Could you check a few things on this model? Use its own coordinates, in mm. Round coordinates to 2 decimals unless told otherwise and drop trailing zeros. Loops run counter-clockwise (first coordinate to the right, second up) from the corner with the lowest first, then second, coordinate; pieces in that order, holes last. Notation, with made-up numbers: (31.5, 44.25) - (63.5, 44.25) arc R29 ccw to (63.5, 66.25) - close; hole circle Ø7 at (70.5, 62). An arc over 180 degrees is marked (long way). Answer as CSV lines item,"result". Start each with the question number.
1) Suppose I cut it at B-B, the plane y = 355.5. Write out the boundary of the cut face in (x, z).
2) Suppose I cut it at C-C, the plane z = 1.2. Count the separate pieces of the cut face and the enclosed holes in it, then the cut area to 3 significant figures.
3) I'm going to push a flat-ended pin straight in: pin 1 Ø3 at (x, y) = (375, 597) entering from +Z. Where does the tip first touch, or does it pass through?
4) Please list where these lines run through material, in increasing order: line 1 along Y through (x, z) = (480, 1.55); line 2 along X through (y, z) = (597, 0.7); line 3 along Y through (x, z) = (155, 1.8).
5) Suppose I cut it at A-A, the plane x = 136.5. Write out the boundary of the cut face in (y, z), then the cut area to 3 significant figures.
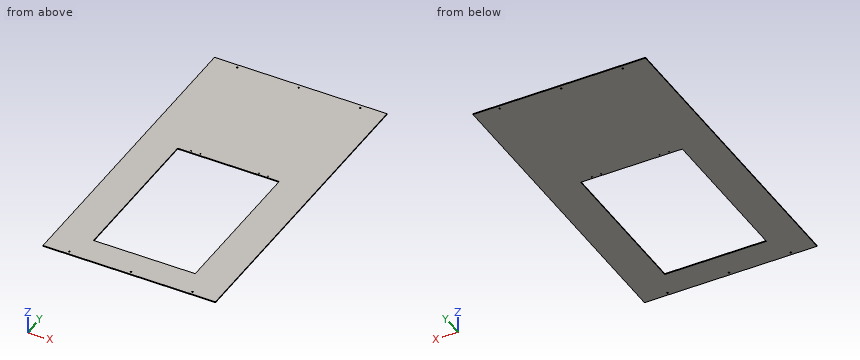
```python
from build123d import *

# Parameters (mm, degrees)
SKETCH_W   = 560
SKETCH_H   = 1020
SKETCH_R   = 2.5
SKETCH_R_2 = 1.6
SKETCH_W_2 = 330
SKETCH_H_2 = 500
PAD_DEPTH  = 3


with BuildPart() as part:
    # Sketch → Pad (new body)
    with BuildSketch(Plane.XY):
        with Locations((280, 510)):
            Rectangle(SKETCH_W, SKETCH_H)
        with Locations((80, 1008)):
            Circle(SKETCH_R, mode=Mode.SUBTRACT)
        with Locations((280, 1008)):
            Circle(SKETCH_R, mode=Mode.SUBTRACT)
        with Locations((480, 1008)):
            Circle(SKETCH_R, mode=Mode.SUBTRACT)
        with Locations((80, 10)):
            Circle(SKETCH_R, mode=Mode.SUBTRACT)
        with Locations((280, 10)):
            Circle(SKETCH_R, mode=Mode.SUBTRACT)
        with Locations((480, 10)):
            Circle(SKETCH_R, mode=Mode.SUBTRACT)
        with Locations((405, 597)):
            Circle(SKETCH_R_2, mode=Mode.SUBTRACT)
        with Locations((155, 597)):
            Circle(SKETCH_R_2, mode=Mode.SUBTRACT)
        with Locations((185, 597)):
            Circle(SKETCH_R_2, mode=Mode.SUBTRACT)
        with Locations((375, 597)):
            Circle(SKETCH_R_2, mode=Mode.SUBTRACT)
        with Locations((280, 340)):
            Rectangle(SKETCH_W_2, SKETCH_H_2, mode=Mode.SUBTRACT)
    extrude(amount=PAD_DEPTH)


solid = part.part
```
Filled sheet:
1,outline,"(0, 0) - (115, 0) - (115, 3) - (0, 3) - close; (445, 0) - (560, 0) - (560, 3) - (445, 3) - close"
2,separate pieces,"1"
2,enclosed holes,"11"
2,area,"406,000 mm²"
3,pin 1,"through"
4,line 1,"0 to 7.5, 12.5 to 1005.5, 1010.5 to 1020"
4,line 2,"0 to 153.4, 156.6 to 183.4, 186.6 to 373.4, 376.6 to 403.4, 406.6 to 560"
4,line 3,"0 to 90, 590 to 595.4, 598.6 to 1020"
5,outline,"(0, 0) - (90, 0) - (90, 3) - (0, 3) - close; (590, 0) - (1020, 0) - (1020, 3) - (590, 3) - close"
5,area,"1,560 mm²"
